Answer from the drawing. Dimensions are ordinates in mm from the lowest x, y and z of the part. Round coordinates to 2 decimals unless told otherwise and drop trailing zeros. Loops run counter-clockwise (first coordinate to the right, second up) from the corner with the lowest first, then second, coordinate; pieces in that order, holes last.
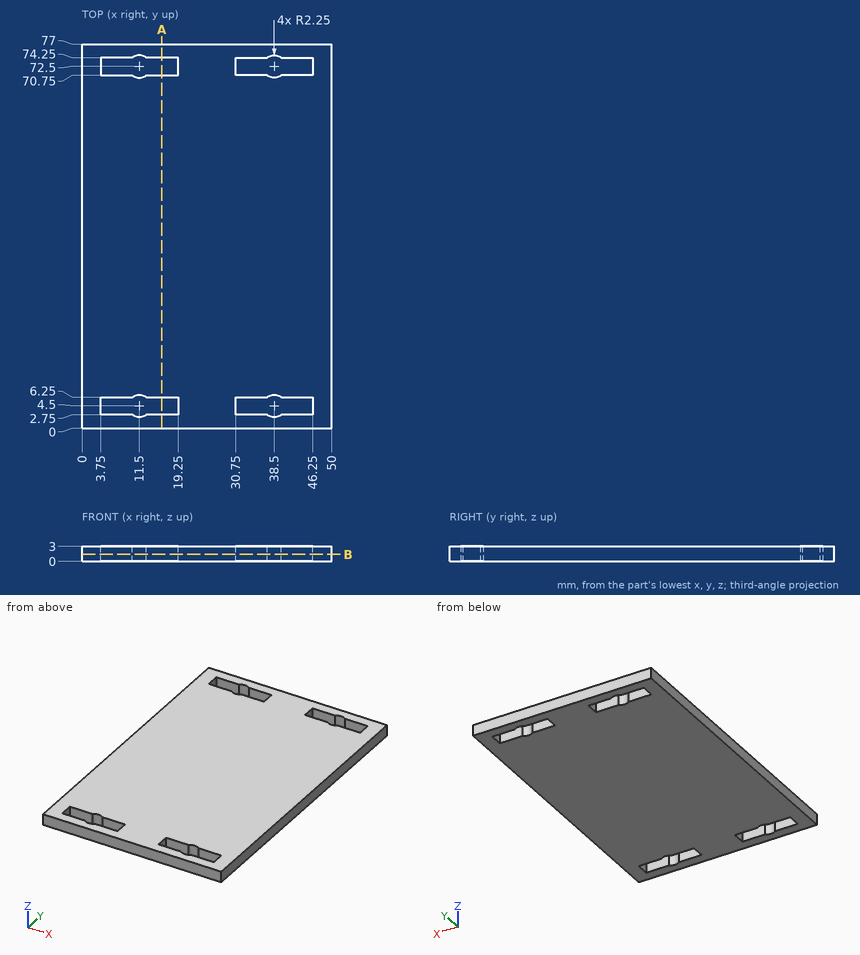
1. Find section B-B (z = 1.4). Give the number of separate pieces and of enclosed holes in the cut face, then the cut area to 3 significant figures.
Answer key:
separate pieces: 1
enclosed holes: 4
area: 3,630 mm2
2. Consider probe 1 along X at (y, z) = (71.5, 1.6); probe 2 along Y at (x, z) = (44.5, 2.45); probe 3 along Y at (x, z) = (37.5, 1.7). Determine where each line is inside the solid, lowest interval first.
Answer key:
probe 1: x = 0 to 3.75, 19.25 to 30.75, 46.25 to 50
probe 2: y = 0 to 2.75, 6.25 to 70.75, 74.25 to 77
probe 3: y = 0 to 2.48, 6.52 to 70.48, 74.52 to 77
3. Find section A-A (x = 16). Write down the section's boundary in (y, z), then the cut area to 3 significant figures.
Answer key:
outline: (0, 0) - (2.75, 0) - (2.75, 3) - (0, 3) - close; (6.25, 0) - (70.75, 0) - (70.75, 3) - (6.25, 3) - close; (74.25, 0) - (77, 0) - (77, 3) - (74.25, 3) - close
area: 210 mm2
